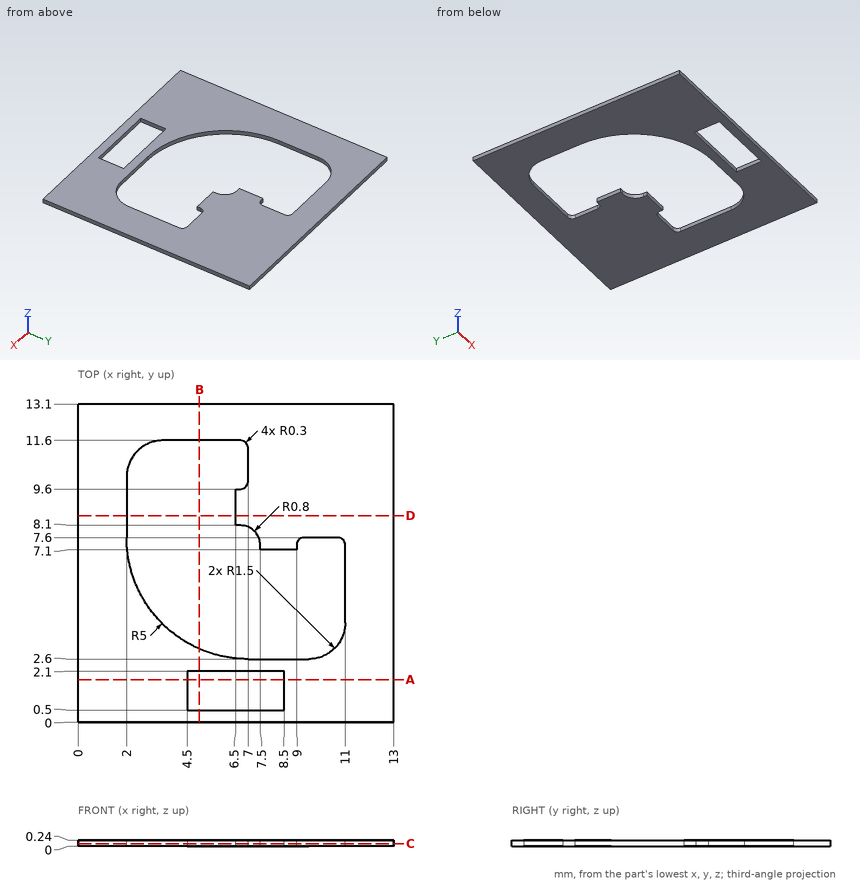
Study the drawing (mm; zero at the part's minimum x, y, z) and answer. Round coordinates to 2 decimals unless told otherwise and drop trailing zeros. Loops run counter-clockwise (first coordinate to the right, second up) from the corner with the lowest first, then second, coordinate; pieces in that order, holes last. Notation, with made-up numbers: (17, 23.5) -> (23, 23.5) arc R14 cw to (23, 37.5) -> close; hole circle Ø1 at (25, 19). An arc over 180 degrees is marked (long way). Use one line per item in the form item = value.
1. The part is cut by section A-A on y = 1.75. Determine the outline of the cut face in (x, z).
Answer key:
outline = (0, 0) -> (4.5, 0) -> (4.5, 0.24) -> (0, 0.24) -> close; (8.5, 0) -> (13, 0) -> (13, 0.24) -> (8.5, 0.24) -> close
2. Find the intervals of material crossed by probe 1 along Y at (x, z) = (8, 0.1); probe 2 along X at (y, z) = (1, 0.1); probe 3 along Y at (x, z) = (4.75, 0.15), in increasing order. Write a range as [from, to].
Answer key:
probe_1 = [0, 0.5], [2.1, 2.6], [7.1, 13.1]
probe_2 = [0, 4.5], [8.5, 13]
probe_3 = [0, 0.5], [2.1, 3.13], [11.6, 13.1]
3. The part is cut by section C-C on z = 0.1. Determine the outline of the cut face in (x, y), and give its area (3 significant figures).
Answer key:
outline = (0, 0) -> (13, 0) -> (13, 13.1) -> (0, 13.1) -> close; hole (2, 7.6) arc R5 ccw to (7, 2.6) -> (9.5, 2.6) arc R1.5 ccw to (11, 4.1) -> (11, 7.3) arc R0.3 ccw to (10.7, 7.6) -> (9.3, 7.6) arc R0.3 ccw to (9, 7.3) -> (9, 7.1) -> (7.5, 7.1) -> (7.5, 7.3) arc R0.8 ccw to (6.7, 8.1) -> (6.5, 8.1) -> (6.5, 9.6) -> (6.7, 9.6) arc R0.3 ccw to (7, 9.9) -> (7, 11.3) arc R0.3 ccw to (6.7, 11.6) -> (3.5, 11.6) arc R1.5 ccw to (2, 10.1) -> close; hole (4.5, 0.5) -> (8.5, 0.5) -> (8.5, 2.1) -> (4.5, 2.1) -> close
area = 107 mm²
4. The part is cut by section B-B on x = 5. Determine the outline of the cut face in (y, z), and give its area (3 significant figures).
Answer key:
outline = (0, 0) -> (0.5, 0) -> (0.5, 0.24) -> (0, 0.24) -> close; (2.1, 0) -> (3.02, 0) -> (3.02, 0.24) -> (2.1, 0.24) -> close; (11.6, 0) -> (13.1, 0) -> (13.1, 0.24) -> (11.6, 0.24) -> close
area = 0.700 mm²
5. The part is cut by section D-D on y = 8.5. Determine the outline of the cut face in (x, z), and give its area (3 significant figures).
Answer key:
outline = (0, 0) -> (2, 0) -> (2, 0.24) -> (0, 0.24) -> close; (6.5, 0) -> (13, 0) -> (13, 0.24) -> (6.5, 0.24) -> close
area = 2.04 mm²
